For this review, take the finished solid that the model builds, in its own axes (mm). Round coordinates to 2 decimals unless told otherwise and drop trailing zeros. Loops run counter-clockwise (first coordinate to the right, second up) from the corner with the lowest first, then second, coordinate; pieces in that order, holes last. Notation, with made-up numbers: (56.5, -26.5) -> (67.5, -26.5) arc R21 ccw to (67.5, 6.5) -> close; hole circle Ø8 at (-10.5, 19). An arc over 180 degrees is marked (long way). Write each question's results on one line, items separated by ' | '.
```python
from build123d import *

# Parameters (mm, degrees)
BOSS_EXTRUDE1_DEPTH      = 3.5
BOSS_EXTRUDE1_DEPTH_BACK = 3.5
SKETCH1_R                = 15
SKETCH1_R_2              = 11


# Read off the part's stored shape, not the designer's step: Cut-Revolve2
with BuildPart() as part:
    # Sketch1 → Boss-Extrude1 (new, two sides: drawn at the far end of the back side and taken through both)
    with BuildSketch(Plane.XY.offset(-BOSS_EXTRUDE1_DEPTH_BACK)):
        Circle(SKETCH1_R)
        Circle(SKETCH1_R_2, mode=Mode.SUBTRACT)
    extrude(amount=BOSS_EXTRUDE1_DEPTH + BOSS_EXTRUDE1_DEPTH_BACK)

    # Cut-Revolve2 outline → Cut-Revolve2 (revolve, cut)
    with BuildSketch(Plane.XZ):
        with BuildLine():
            ThreePointArc((14.120311353, 3.5), (14.712206017, 3.212206017), (15, 2.620311353))
            Line((15, 2.620311353), (15, 3.5))
            Line((15, 3.5), (14.120311353, 3.5))
        make_face()
        with BuildLine():
            Line((15, -2.379688647), (15, 2.379688647))
            ThreePointArc((15, 2.379688647), (14.789015345, 1.873957185), (14.34448659, 1.553530872))
            Line((14.34448659, 1.553530872), (12.657979857, 0.939692621))
            ThreePointArc((12.657979857, 0.939692621), (12, 0), (12.657979857, -0.939692621))
            Line((12.657979857, -0.939692621), (14.34448659, -1.553530872))
            ThreePointArc((14.34448659, -1.553530872), (14.789015345, -1.873957185), (15, -2.379688647))
        make_face()
        with BuildLine():
            Line((15, -3.5), (15, -2.620311353))
            ThreePointArc((15, -2.620311353), (14.712206017, -3.212206017), (14.120311353, -3.5))
            Line((14.120311353, -3.5), (15, -3.5))
        make_face()
    revolve(axis=Axis((0, 0, 0), (0, 0, 1)), mode=Mode.SUBTRACT)


solid = part.part
```
1. Consider section C-C (z = -0.5). State the section outline as (x, y) points.
Values found:
outline: circle Ø24.27 at (0, 0); hole circle Ø22 at (0, 0)
2. To check wall thickness, follow probe 1 along Y at (x, z) = (0, -0.25); probe 2 along X at (y, z) = (5.25, 3); probe 3 along Z at (x, y) = (-4.75, 13.75). State the ranges of each line that lie inside material, in increasing order.
Values found:
probe 1: y = -12.03 to -11, 11 to 12.03 | probe 2: x = -13.92 to -9.67, 9.67 to 13.92 | probe 3: z = -3.35 to -1.65, 1.65 to 3.35
3. For pin 1 (3 mm diameter, centred on x = 10.5, z = -0.5, fed in from -Y); pin 2 (1.5 mm diameter, centred on y = 7, z = -2, fed in from +X); pin 3 (4 mm diameter, centred on y = 1.5, z = 1, fed in from -X); pin 4 (1 mm diameter, centred on y = 7, z = 2.5, fed in from -X), all flat-tipped, find the tip position at first contact; note any pin that passes through.
Values found:
pin 1: stops at y = -11.04 | pin 2: stops at x = 13.59 | pin 3: stops at x = -15 | pin 4: stops at x = -13.52
4. Consider section A-A (y = 0). State the section outline as (x, z) points.
Values found:
outline: (-15, -2.62) arc R1.01 ccw to (-14.12, -3.5) -> (-11, -3.5) -> (-11, 3.5) -> (-14.12, 3.5) arc R1.01 ccw to (-15, 2.62) -> (-15, 2.38) arc R1.01 ccw to (-14.34, 1.55) -> (-12.66, 0.94) arc R1 cw to (-12.66, -0.94) -> (-14.34, -1.55) arc R1.01 ccw to (-15, -2.38) -> close; (11, -3.5) -> (14.12, -3.5) arc R1.01 ccw to (15, -2.62) -> (15, -2.38) arc R1.01 ccw to (14.34, -1.55) -> (12.66, -0.94) arc R1 cw to (12.66, 0.94) -> (14.34, 1.55) arc R1.01 ccw to (15, 2.38) -> (15, 2.62) arc R1.01 ccw to (14.12, 3.5) -> (11, 3.5) -> close
